```python
from build123d import *

# Parameters (mm, degrees)
SKETCH1_W           = 153
SKETCH1_H           = 134.8
BOSS_EXTRUDE1_DEPTH = 85.2
SHELL1_T            = -1.5
SKETCH2_W           = 85.2
SKETCH2_H           = 134.8
CUT_EXTRUDE1_DEPTH  = 1.5
SKETCH3_W           = 151.5
SKETCH3_H           = 134.8
CUT_EXTRUDE2_DEPTH  = 1.5


with BuildPart() as part:
    # Sketch1 → Boss-Extrude1 (new body)
    with BuildSketch(Plane.YZ):
        with Locations((76.5, 67.4)):
            Rectangle(SKETCH1_W, SKETCH1_H)
    extrude(amount=BOSS_EXTRUDE1_DEPTH)

    # Shell1
    shell1_openings = [part.faces().sort_by_distance(p)[0] for p in [
        (42.6, 76.5, 0),
    ]]
    offset(amount=SHELL1_T, openings=shell1_openings, kind=Kind.INTERSECTION)

    # Sketch2 → Cut-Extrude1 (cut)
    with BuildSketch(Plane.XZ):
        with Locations((42.6, 67.4)):
            Rectangle(SKETCH2_W, SKETCH2_H)
    extrude(amount=-CUT_EXTRUDE1_DEPTH, mode=Mode.SUBTRACT)

    # Sketch3 → Cut-Extrude2 (cut)
    with BuildSketch(Plane(origin=(0, 0, 0), x_dir=(0, -1, 0), z_dir=(-1, 0, 0))):
        with Locations((-77.25, 67.4)):
            Rectangle(SKETCH3_W, SKETCH3_H)
    extrude(amount=-CUT_EXTRUDE2_DEPTH, mode=Mode.SUBTRACT)


solid = part.part
```
Design review of the part built by this model. Coordinates are the model's own, in mm. A direction names the side the tool comes from. Give positions to 0.01 mm unless a question says otherwise; leave off trailing zeros. Write each loop counter-clockwise with the first axis right and the second up, starting at its lowest first coordinate (ties: lowest second). Pieces come first, ordered by that corner, then holes. Notation, with made-up numbers: (-16, -12.75) -> (27, -12.75) arc R12 cw to (27, 7.25) -> close; hole circle Ø8 at (84.25, 23). An arc over 180 degrees is marked (long way). Answer in a Markdown table with one row per item.
(1) To check wall thickness, follow probe 1 along X at (y, z) = (110, 106.5); probe 2 along Z at (x, y) = (40.5, 41); probe 3 along Y at (x, z) = (73, 81.5). State the ranges of each line that lie inside material, in increasing order.
Results:
| item | result |
|---|---|
| probe 1 | 83.7 to 85.2 |
| probe 2 | 133.3 to 134.8 |
| probe 3 | 151.5 to 153 |
(2) Consider section A-A (x = 29.5). State the section outline as (y, z) points, then the cut area to 3 significant figures.
Results:
| item | result |
|---|---|
| outline | (1.5, 133.3) -> (151.5, 133.3) -> (151.5, 0) -> (153, 0) -> (153, 134.8) -> (1.5, 134.8) -> close |
| area | 427 mm2 |
(3) Clearance check with flat-ended pins moving along their axes: pin 1 (2 mm diameter, centred on x = 54, z = 90, fed in from -Y); pin 2 (6 mm diameter, centred on y = 69, z = 22.5, fed in from -X); pin 3 (4 mm diameter, centred on x = 61.5, y = 62.5, fed in from -Z). State where each tip first meets the part, or that it passes through.
Results:
| item | result |
|---|---|
| pin 1 | y = 151.5 |
| pin 2 | x = 83.7 |
| pin 3 | z = 133.3 |
(4) Consider section B-B (z = 58). State the section outline as (x, y) points.
Results:
| item | result |
|---|---|
| outline | (1.5, 151.5) -> (83.7, 151.5) -> (83.7, 1.5) -> (85.2, 1.5) -> (85.2, 153) -> (1.5, 153) -> close |
(5) For faces 1 (the flat face through (42, 75, 133.3)), 2 (the flat face through (85.2, 76, 68)), list the 3-axis set-ups (+Z, -Z, +X, -X, +Y, -Y) from which the entire face can be reached by the end or side of a thin tool; tool diameter is ignored.
Results:
| item | result |
|---|---|
| face 1 | -Z, -X, -Y |
| face 2 | +Z, -Z, +X, +Y, -Y |
